Verification items for the finished model (mm, model axes). Round coordinates to 2 decimals unless told otherwise and drop trailing zeros. Write each loop counter-clockwise with the first axis right and the second up, starting at its lowest first coordinate (ties: lowest second). Pieces come first, ordered by that corner, then holes. Notation, with made-up numbers: M 77.5,-39.5 L 103.5,-39.5 A12 cw 103.5,-24.5 Z; hole C 81.25,-12 d9. An arc over 180 degrees is marked long. One line per question, with ' | ' between items.
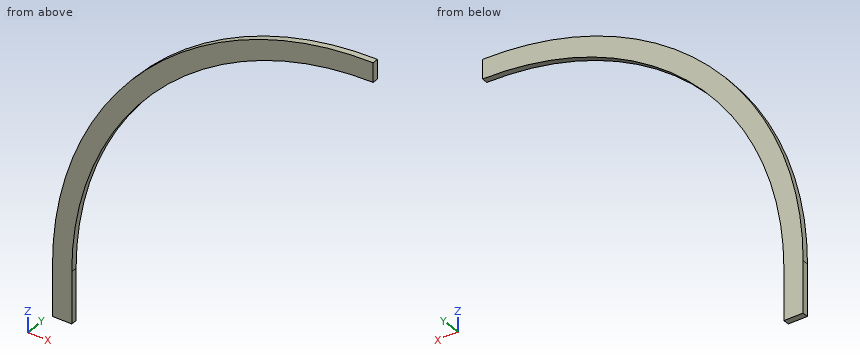
from build123d import *

# Parameters (mm, degrees)
BOSS_EXTRUDE1_DEPTH = 9.525
SKETCH3_W           = 30
SKETCH3_H           = 9.525
BOSS_EXTRUDE2_DEPTH = 80


with BuildPart() as part:
    # Sketch2 → Boss-Extrude1 (new body)
    with BuildSketch(Plane(origin=(0, 0, 0), x_dir=(1, 0, 0), z_dir=(0, 1, 0))):
        with BuildLine():
            ThreePointArc((0, -470), (-332.340187158, -332.340187158), (-470, 0))
            Line((-470, 0), (-500, 0))
            ThreePointArc((-500, 0), (-353.553390593, -353.553390593), (0, -500))
            Line((0, -500), (0, -470))
        make_face()
    extrude(amount=BOSS_EXTRUDE1_DEPTH)

    # Sketch3 → Boss-Extrude2 (add)
    with BuildSketch(Plane(origin=(0, 0, 0), x_dir=(-1, 0, 0), z_dir=(0, 0, -1))):
        with Locations((485, 4.7625)):
            Rectangle(SKETCH3_W, SKETCH3_H)
    extrude(amount=BOSS_EXTRUDE2_DEPTH)


solid = part.part
1. Section check B-B, the plane z = -9. Record the cut outline in (x, y) (3 decimals), then the cut area to 3 significant figures.
Results:
outline: M -500,0 L -470,0 L -470,9.525 L -500,9.525 Z | area: 286 mm2
2. Thickness scan on line 1 (X direction, y = 1.75, z = -20); line 2 (Z direction, x = -388, y = 4.25); line 3 (Z direction, x = -358, y = 8.5). Record the ranges inside material, lowest first.
Results:
line 1: x = -500 to -470 | line 2: z = 265.25 to 315.37 | line 3: z = 304.53 to 349.05
3. Go/stop test with flat-tipped pins: P1, Ø1.5, axis at x = -357, y = 6.5, coming from the -Z side; P2, Ø5, axis at x = -158, y = 7, coming from the -Z side; P3, Ø2, axis at x = -365, y = 3, coming from the +Z side. Record where each tip stops, or that it passes through.
Results:
P1: stops at z = 304.82 | P2: stops at z = 441.75 | P3: stops at z = 342.79
4. Section check A-A, the plane y = 8. Record the cut outline in (x, z), then the cut area to 3 significant figures.
Results:
outline: M -500,-80 L -470,-80 L -470,0 A470 cw 0,470 L 0,500 A500 ccw -500,0 Z | area: 25,300 mm2
5. Section check C-C, the plane x = -219. Record the cut outline in (y, z) (3 decimals).
Results:
outline: M 0,415.859 L 9.525,415.859 L 9.525,449.487 L 0,449.487 Z
